Autodesk Inventor part; units mm, degrees
ref_plane "Work Plane1" through (0, 0, 16) normal (0, 0, 1) x (1, 0, 0)
ref_plane "YZ Plane" through (0, 0, 0) normal (1, 0, 0) x (0, 1, 0)
ref_plane "XZ Plane" through (0, 0, 0) normal (0, 1, 0) x (-1, 0, 0)
sketch "Sketch1" plane through (0, 0, 0) normal (0, 0, 1) x (1, 0, 0)
  line L0 (0, 0) -> (5.038, 40.6155)
  circle A0 centre (10, 40) radius 5
  line L1 (14.962, 40.6155) -> (20, 0)
  line L2 (20, 0) -> (0, 0)
  circle A1 centre (10, 40) radius 2.5
  line L3 (2.5, 0) -> (2.5, 20.1545)
  line L4 (17.5, 0) -> (17.5, 20.1545)
  dimension "d0" = 5
  dimension "d1" = 10
  dimension "d2" = 20
  dimension "d3" = 10
  dimension "d4" = 40
  dimension "d19" = 15
  dimension "d20" = 7.5
extrude "Extrusion1" add sketch "Sketch1" along normal blind 32
ref_plane "Work Plane1" through (0, 0, 16) normal (0, 0, 1) x (1, 0, 0)
sketch "Sketch2" plane through (0, 0, 16) normal (0, 0, 1) x (1, 0, 0)
  circle A0 centre (10, 40) radius 2.5
  arc A1 (14.962, 40.6155) -> (5.038, 40.6155) centre (10, 40) ccw
  line L0 (20, 0) -> (14.962, 40.6155)
  line L1 (0, 0) -> (20, 0)
  line L2 (5.038, 40.6155) -> (0, 0)
  line L3 (1.8606, 52.4259) -> (18.1394, 52.4259)
  line L4 (18.1394, 52.4259) -> (18.1394, 15)
  line L5 (18.1394, 15) -> (1.8606, 15)
  line L6 (1.8606, 15) -> (1.8606, 52.4259)
  dimension "d21" = 25
extrude "Extrusion2" cut sketch "Sketch2" along normal mid plane 19 contours A0 | L0 L5 L2 A1 | A1 L2 L6 L3 L4 L0
sketch "Sketch3" plane through (0, 0, 0) normal (0, -1, 0) x (1, 0, 0)
  line L0 (0, 0) -> (20, 0)
  line L1 (20, 0) -> (20, 32)
  line L2 (0, 32) -> (20, 32)
  line L3 (0, 0) -> (0, 32)
  circle A0 centre (10, 16) radius 4.7625
  dimension "d14" = 9.525
  dimension "d15" = 10
  dimension "d16" = 16
extrude "Extrusion3" cut sketch "Sketch3" against normal up to next contours A0
fillet "Fillet1" radius 2 2 edges at (10, 15, 6.5) (10, 15, 25.5)
sketch "Sketch5" plane through (0, 0, 32) normal (0, 0, 1) x (1, 0, 0)
  line L0 (0, 0) -> (2, 0)
  line L1 (0, 0) -> (20, 0)
  line L2 (2, 0) -> (2, 16.1236)
  line L3 (5.038, 40.6155) -> (0, 0)
  line L4 (2, 16.1236) -> (0, 0)
  line L5 (0, 0) -> (0, 22.2881)
  line L6 (20, 0) -> (18, 0)
  line L7 (18, 0) -> (18, 16.1236)
  line L8 (18, 16.1236) -> (20, 0)
  line L9 (20, 0) -> (14.962, 40.6155)
  dimension "d27" = 2
  dimension "d28" = 2
extrude "Extrusion5" cut sketch "Sketch5" against normal up to next
properties part number "hinge_for_swing" material "Acetal Resin, Black"
The listing builds one solid part. Answer for the finished solid, in the listing's coordinates (mm). A direction names the side the tool comes from. Coordinates: 2 decimals unless noted, no trailing zeros. Write each loop counter-clockwise with the first axis right and the second up, starting at its lowest first coordinate (ties: lowest second). Pieces come first, ordered by that corner, then holes. Notation, with made-up numbers: (46, 60) -> (61, 60) arc R15 ccw to (61, 89) -> close; hole circle Ø4 at (86.25, -12.5). An arc over 180 degrees is marked (long way). One line per question, with ' | ' between items.
1. Which of the six approach directions +Z, -Z, +X, -X, +Y, -Y give full straight-line access (tool end or side, diameter ignored) to faces 1 (the flat face through (10, 28, 6.5)), 2 (the cylindrical face through (10, 45, 3))?
Verdict:
face 1: +X, -X, +Y | face 2: +Z, -Z, +Y
2. Section D-D (y = 4) is taken. Determine the outline of the cut face in (x, z) (1 decimal).
Verdict:
outline: (2, 0) -> (18, 0) -> (18, 32) -> (2, 32) -> close; hole circle Ø9.5 at (10, 16)
3. Section B-B (x = 10) is taken. Determine the outline of the cut face in (y, z), and give its area (3 significant figures).
Verdict:
outline: (0, 0) -> (37.5, 0) -> (37.5, 6.5) -> (17, 6.5) arc R2 cw to (15, 8.5) -> (15, 11.24) -> (0, 11.24) -> close; (0, 20.76) -> (15, 20.76) -> (15, 23.5) arc R2 cw to (17, 25.5) -> (37.5, 25.5) -> (37.5, 32) -> (0, 32) -> close; (42.5, 0) -> (45, 0) -> (45, 6.5) -> (42.5, 6.5) -> close; (42.5, 25.5) -> (45, 25.5) -> (45, 32) -> (42.5, 32) -> close | area: 664 mm^2
4. Section A-A (z = 16) is taken. Determine the outline of the cut face in (x, y), and give its area (3 significant figures).
Verdict:
outline: (2, 0) -> (5.24, 0) -> (5.24, 15) -> (2, 15) -> close; (14.76, 0) -> (18, 0) -> (18, 15) -> (14.76, 15) -> close | area: 97.1 mm^2
5. For a pull along Y with two mould halves and no side action, classify faces 3 (the flat face through (16.46, 28.54, 3.3)), 4 (the cylindrical face through (9.46, 42.44, 28.7)), 5 (the flat face through (10, 23, 32)) as released by +Y, released by -Y, zero draft, split by the parting line, or undercut.
Verdict:
face 3: released by +Y | face 4: undercut | face 5: zero draft
6. Given pin 1 Ø4.5 at (x, y) = (10, 40) entering from -Z; pin 2 Ø1.5 at (y, z) = (21.5, 5) entering from +X; pin 3 Ø1.5 at (x, z) = (4, 22.5) entering from +Y, each flat-ended and moving along its own axis, determine where each tip first touches the part or whether it passes through.
Verdict:
pin 1: passes through | pin 2: stops at x = 17.43 | pin 3: stops at y = 15
7. Straight lines are drawn through the part: line 1 (Z direction, x = 12.25, y = 25); line 2 (Z direction, x = 10, y = 9); line 3 (Y direction, x = 10, z = 2.5). For each, find the intervals that lie inside material, in ascending order.
Verdict:
line 1: z = 0 to 6.5, 25.5 to 32 | line 2: z = 0 to 11.24, 20.76 to 32 | line 3: y = 0 to 37.5, 42.5 to 45
8. Section C-C (y = 31) is taken. Determine the outline of the cut face in (x, z).
Verdict:
outline: (3.85, 0) -> (16.15, 0) -> (16.15, 6.5) -> (3.85, 6.5) -> close; (3.85, 25.5) -> (16.15, 25.5) -> (16.15, 32) -> (3.85, 32) -> close
